Can you work these out from the drawing? Everything is in mm from the part's minimum corner. A direction names the side the tool comes from. Round coordinates to 2 decimals unless told otherwise and drop trailing zeros. Write each loop counter-clockwise with the first axis right and the second up, starting at its lowest first coordinate (ties: lowest second). Pieces come first, ordered by that corner, then holes. Notation, with made-up numbers: M 52.25,-7.5 L 99.25,-7.5 A11 ccw 99.25,-3.5 Z; hole C 49,52.25 d11. An arc over 180 degrees is marked long. Answer in a Markdown table with one row per item. Add a question column.
(1) I'm going to push flat-ended pins straight in: pin 1 (2 mm diameter, centred on x = 30.5, z = 7.5, fed in from -Y); pin 2 (1.5 mm diameter, centred on y = 122, z = 8.5, fed in from +X); pin 3 (2 mm diameter, centred on x = 38.5, y = 174.92, fed in from +Z); pin 4 (10 mm diameter, centred on y = 115.5, z = 9, fed in from -X). Where does each tip first touch, or does it pass through?
(2) If we mould it in two halves opening along X, with no side actions, what happens to the marked faces 3, 4 and 5? For each: released by +X, released by -X, zero draft, split by the parting line, or undercut.
(3) If I drill on probe 1 along Y at (x, z) = (23.5, 0.9); probe 2 along Y at (x, z) = (38.5, 18); probe 3 along X at (y, z) = (32, 11.25), over which ranges is the centre line in solid material (lowest first)?
(4) For the marked faces 1 and 2, which set-ups out of +Z, -Z, +X, -X, +Y, -Y let a thin tool reach every point of the face, with its end or its side?
(5) Suppose I cut it at D-D, the plane y = 154.5. Write out the boundary of the cut face in (x, z).
(6) Suppose I cut it at B-B, the plane x = 23.5. Write out the boundary of the cut face in (y, z).
(7) Suppose I cut it at A-A, the plane y = 10. Write out the boundary of the cut face in (x, z).
(8) Suppose I cut it at C-C, the plane z = 5.5. Write out the boundary of the cut face in (x, y).
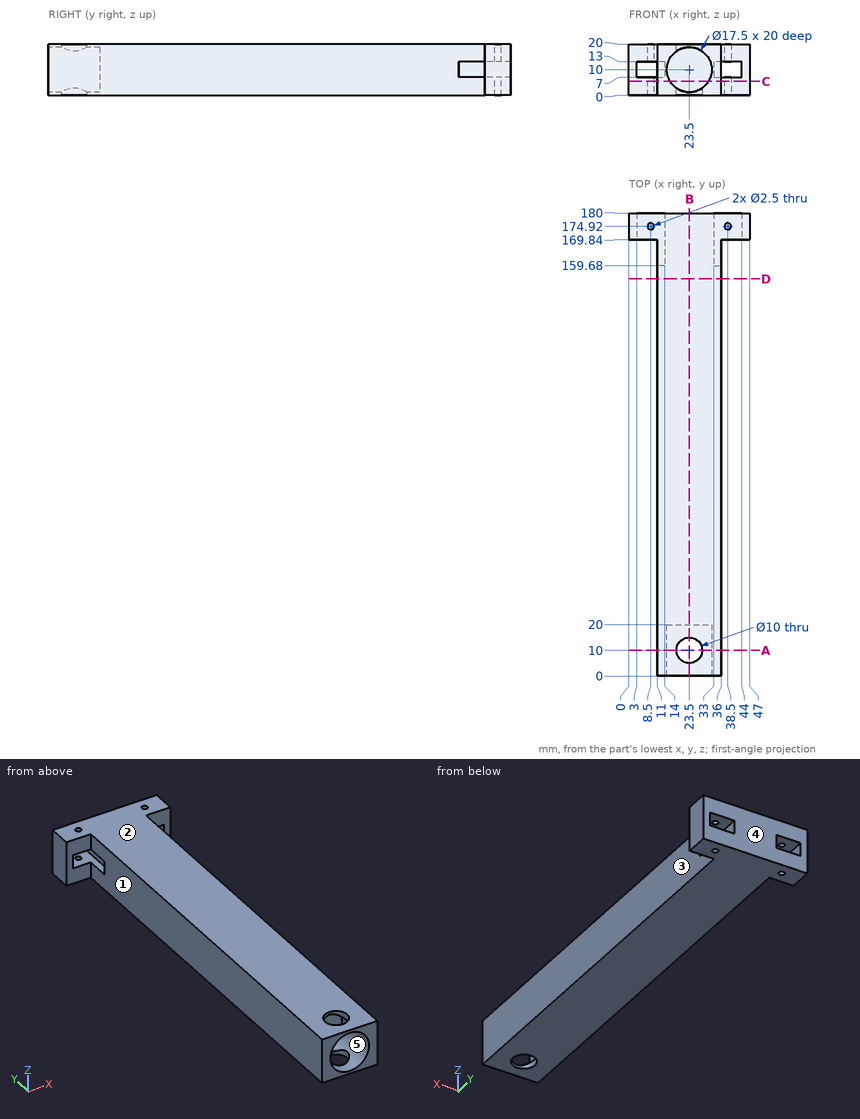
Calculated:
| question | item | result |
|---|---|---|
| 1 | pin 1 | y = 20 |
| 1 | pin 2 | x = 36 |
| 1 | pin 3 | through |
| 1 | pin 4 | x = 11 |
| 2 | face 3 | released by +X |
| 2 | face 4 | zero draft |
| 2 | face 5 | undercut |
| 3 | probe 1 | 0 to 5, 15 to 180 |
| 3 | probe 2 | 169.84 to 173.67, 176.17 to 180 |
| 3 | probe 3 | 11 to 36 |
| 4 | face 1 | +Z, -Z, -X, -Y |
| 4 | face 2 | +Z, +X, -X, +Y, -Y |
| 5 | outline | M 11,0 L 36,0 L 36,20 L 11,20 Z |
| 6 | outline | M 0,0 L 5,0 L 5,1.25 L 0,1.25 Z; M 0,18.75 L 5,18.75 L 5,20 L 0,20 Z; M 15,0 L 180,0 L 180,20 L 15,20 L 15,18.75 L 20,18.75 L 20,1.25 L 15,1.25 Z |
| 7 | outline | M 11,0 L 18.5,0 L 18.5,2.82 A8.75 cw 18.5,17.18 L 18.5,20 L 11,20 Z; M 28.5,0 L 36,0 L 36,20 L 28.5,20 L 28.5,17.18 A8.75 cw 28.5,2.82 Z |
| 8 | outline | M 0,169.84 L 11,169.84 L 11,0 L 16,0 L 16,20 L 31,20 L 31,0 L 36,0 L 36,169.84 L 47,169.84 L 47,180 L 0,180 Z; hole C 8.5,174.92 d2.5; hole C 38.5,174.92 d2.5 |
